Design review of the part built by this model. Coordinates are the model's own, in mm. Face numbers are marked on the shaded views. A direction names the side the tool comes from. Coordinates: 2 decimals unless noted, no trailing zeros. Write each loop counter-clockwise with the first axis right and the second up, starting at its lowest first coordinate (ties: lowest second). Pieces come first, ordered by that corner, then holes. Notation, with made-up numbers: (16, 56.25) - (42, 56.25) arc R20 cw to (42, 76.25) - close; hole circle Ø6 at (51, 63). An arc over 180 degrees is marked (long way). Answer as a JSON object with one key per item and string values.
```python
from build123d import *

# Parameters (mm, degrees)
SKETCH1_W           = 210
SKETCH1_H           = 136
SKETCH1_W_2         = 200
SKETCH1_H_2         = 126
EXTRUDE_THIN1_DEPTH = 50
SKETCH1_2_W         = 200
SKETCH1_2_H         = 126
BOSS_EXTRUDE1_DEPTH = 5
FILLET1_R           = 5
SKETCH2_W           = 202
SKETCH2_H           = 5
CUT_EXTRUDE1_DEPTH  = 133
SKETCH3_W           = 17
SKETCH3_H           = 15
SKETCH3_W_2         = 10
SKETCH3_H_2         = 10
CUT_EXTRUDE2_DEPTH  = 10


with BuildPart() as part:
    # Sketch1 → Extrude-Thin1 (new body)
    with BuildSketch(Plane(origin=(0, 0, 0), x_dir=(1, 0, 0), z_dir=(0, 1, 0))):
        with Locations((100, 63)):
            Rectangle(SKETCH1_W, SKETCH1_H)
        with Locations((100, 63)):
            Rectangle(SKETCH1_W_2, SKETCH1_H_2, mode=Mode.SUBTRACT)
    extrude(amount=EXTRUDE_THIN1_DEPTH)

    # Sketch1<2> → Boss-Extrude1 (add)
    with BuildSketch(Plane(origin=(0, 0, 0), x_dir=(1, 0, 0), z_dir=(0, 1, 0))):
        with Locations((100, 63)):
            Rectangle(SKETCH1_2_W, SKETCH1_2_H)
    extrude(amount=BOSS_EXTRUDE1_DEPTH)

    # Fillet1
    fillet1_edges = [part.edges().sort_by_distance(p)[0] for p in [
        (100, 0, -131),
        (205, 0, -63),
        (100, 0, 5),
        (-5, 0, -63),
        (-5, 25, -131),
        (205, 25, -131),
        (205, 25, 5),
        (-5, 25, 5),
    ]]
    fillet(fillet1_edges, radius=FILLET1_R)

    # Sketch2 → Cut-Extrude1 (cut)
    with BuildSketch(Plane.XY.offset(5)):
        with Locations((100, 44.5)):
            Rectangle(SKETCH2_W, SKETCH2_H)
    extrude(amount=-CUT_EXTRUDE1_DEPTH, mode=Mode.SUBTRACT)

    # Sketch3 → Cut-Extrude2 (cut)
    with BuildSketch(Plane(origin=(205, 0, 0), x_dir=(0, 0, -1), z_dir=(1, 0, 0))):
        with Locations((15.19, 19.17)):
            Rectangle(SKETCH3_W, SKETCH3_H)
        with Locations((35.51, 19.17)):
            Rectangle(SKETCH3_W, SKETCH3_H)
        with Locations((55.83, 19.17)):
            Rectangle(SKETCH3_W, SKETCH3_H)
        with Locations((76.15, 19.17)):
            Rectangle(SKETCH3_W, SKETCH3_H)
        with Locations((113.435, 16.67)):
            Rectangle(SKETCH3_W_2, SKETCH3_H_2)
    extrude(amount=-CUT_EXTRUDE2_DEPTH, mode=Mode.SUBTRACT)


solid = part.part
```
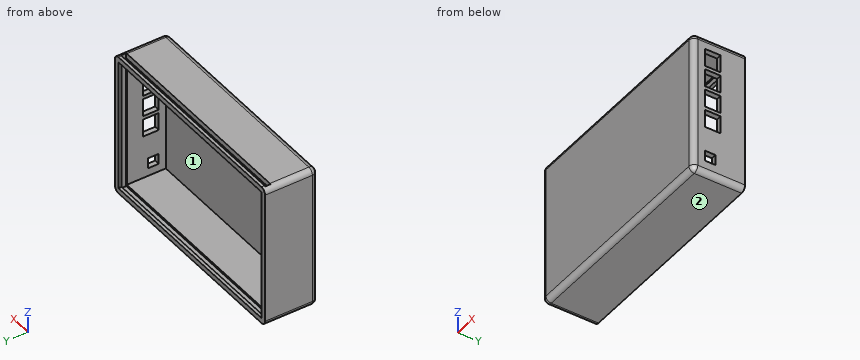
(1) For pin 1 (1.5 mm diameter, centred on x = 203.5, y = 20.5, fed in from -Z); pin 2 (4 mm diameter, centred on x = 148, z = -16, fed in from +Y); pin 3 (5 mm diameter, centred on y = 21.5, z = -58, fed in from +X); pin 4 (4 mm diameter, centred on x = 201.5, y = 21, fed in from -Z), all flat-tipped, find the tip position at first contact; note any pin that passes through.
Solved:
{"pin 1": "stops at z = -130.18", "pin 2": "stops at y = 5", "pin 3": "stops at x = 0", "pin 4": "stops at z = -131"}
(2) Take a section at C-C, the plane y = 7.5. Write out the cut boundary in (x, z), and give its area (3 significant figures).
Solved:
{"outline": "(-5, -126) arc R5 ccw to (0, -131) - (200, -131) arc R5 ccw to (205, -126) - (205, 0) arc R5 ccw to (200, 5) - (0, 5) arc R5 ccw to (-5, 0) - close; hole (0, -126) - (200, -126) - (200, 0) - (0, 0) - close", "area": "3,340 mm^2"}
(3) To check wall thickness, follow line 1 (X direction, y = 17, z = -96); line 2 (Z direction, x = 181.5, y = 27); line 3 (Y direction, x = 148, z = -98). State the ranges of each line that lie inside material, in increasing order. Write a range as from..to.
Solved:
{"line 1": "x = -5..0, 200..205", "line 2": "z = -131..-126, 0..5", "line 3": "y = 0..5"}
(4) Tool access review of the marked faces 1 and 2: name each direction out of +Z, -Z, +X, -X, +Y, -Y from which nothing blocks a thin tool from reaching the whole face with its end or side.
Solved:
{"face 1": "+Y", "face 2": "-Z, +X, -X, +Y, -Y"}
(5) Take a section at B-B, the plane x = 129. Write out the cut boundary in (y, z).
Solved:
{"outline": "(0, -126) arc R5 ccw to (5, -131) - (50, -131) - (50, -126) - (47, -126) - (47, -128) - (42, -128) - (42, -126) - (5, -126) - (5, 0) - (42, 0) - (42, 5) - (5, 5) arc R5 ccw to (0, 0) - close; (47, 0) - (50, 0) - (50, 5) - (47, 5) - close"}
(6) Take a section at D-D, the plane y = 17. Give the number of separate pieces and of enclosed holes in the cut face, and give its area (3 significant figures).
Solved:
{"separate pieces": "5", "enclosed holes": "0", "area": "2,950 mm^2"}
(7) Take a section at A-A, the plane z = -19.5. Write out the cut boundary in (x, y).
Solved:
{"outline": "(-5, 5) arc R5 ccw to (0, 0) - (200, 0) arc R5 ccw to (205, 5) - (205, 11.67) - (200, 11.67) - (200, 5) - (0, 5) - (0, 42) - (-1, 42) - (-1, 47) - (0, 47) - (0, 50) - (-5, 50) - close; (200, 26.67) - (205, 26.67) - (205, 50) - (200, 50) - (200, 47) - (201, 47) - (201, 42) - (200, 42) - close"}
